from build123d import *

# Parameters (mm, degrees)
SKETCH_1_R               = 7
EXTRUDE_1_DEPTH          = 4
SKETCH_2_R               = 7
EXTRUDE_2_DEPTH          = 30
SKETCH_4_R               = 1
SKETCH_4_R_2             = 0.5
EXTRUDE_3_DEPTH          = 8
EXTRUDE_4_DEPTH          = 4
CUT_EXTRUDE_1_DEPTH      = 4
EXTRUDE_5_DEPTH          = 12
EXTRUDE_5_DEPTH_BACK     = 12
SKETCH_9_R               = 8.062257748
SKETCH_12_R              = 5
CUT_EXTRUDE_2_DEPTH      = 10
CUT_EXTRUDE_3_DEPTH      = 49.277651166
CUT_EXTRUDE_3_DEPTH_BACK = 49.277651166
SKETCH_13_R              = 1.5


with BuildPart() as part:
    # 草图1 → 凸台-拉伸1 (new body)
    with BuildSketch(Plane(origin=(0, 0, 0), x_dir=(1, 0, 0), z_dir=(0, 1, 0))):
        with Locations(Location((0, 0, 0), (0, 0, 270))):
            Circle(SKETCH_1_R)
    extrude(amount=EXTRUDE_1_DEPTH)

    # 草图2 → 凸台-拉伸2 (add)
    with BuildSketch(Plane(origin=(0, 4, 0), x_dir=(1, 0, 0), z_dir=(0, 1, 0))):
        with Locations(Location((0, 0, 0), (0, 0, 270))):
            Circle(SKETCH_2_R)
    extrude(amount=EXTRUDE_2_DEPTH)

    # 草图4 → 凸台-拉伸3 (add)
    with BuildSketch(Plane(origin=(0, 34, 0), x_dir=(1, 0, 0), z_dir=(0, 1, 0))):
        with Locations((5.663466382, -4.114018539)):
            Circle(SKETCH_4_R)
        with Locations((5.663466382, -4.114018539)):
            Circle(SKETCH_4_R_2, mode=Mode.SUBTRACT)
    extrude(amount=-EXTRUDE_3_DEPTH)

    # 草图5 → 凸台-拉伸4 (add)
    with BuildSketch(Plane(origin=(0, 21, 0), x_dir=(-1, 0, 0), z_dir=(0, -1, 0))):
        with BuildLine():
            ThreePointArc((-5.355347766, -4.507798831), (-5.190723909, -4.696422606), (-5.01946017, -4.879038799))
            ThreePointArc((-5.01946017, -4.879038799), (-6.472533008, -4.701735473), (-6.191891648, -3.265038717))
            ThreePointArc((-6.191891648, -3.265038717), (-6.071173774, -3.484372111), (-5.942689761, -3.699248356))
            ThreePointArc((-5.942689761, -3.699248356), (-6.067999695, -4.407877006), (-5.355347766, -4.507798831))
        make_face()
    extrude(amount=EXTRUDE_4_DEPTH)

    # 草图10 → 切除-拉伸1 (cut)
    with BuildSketch(Plane(origin=(0, 34, 0), x_dir=(1, 0, 0), z_dir=(0, 1, 0))):
        with BuildLine():
            ThreePointArc((5.355347766, -4.507798831), (6.067999695, -4.407877006), (5.942689761, -3.699248356))
            ThreePointArc((5.942689761, -3.699248356), (6.071173774, -3.484372111), (6.191891648, -3.265038717))
            ThreePointArc((6.191891648, -3.265038717), (6.472533008, -4.701735473), (5.01946017, -4.879038799))
            ThreePointArc((5.01946017, -4.879038799), (5.190723909, -4.696422606), (5.355347766, -4.507798831))
        make_face()
    extrude(amount=-CUT_EXTRUDE_1_DEPTH, mode=Mode.SUBTRACT)

    # 草图9 → 凸台-拉伸5 (add, two sides: drawn at the far end of the back side and taken through both)
    with BuildSketch(Plane(origin=(0, 0, 0), x_dir=(0, 0, -1), z_dir=(1, 0, 0)).offset(-EXTRUDE_5_DEPTH_BACK)):
        with Locations((0, 38)):
            Circle(SKETCH_9_R)
    extrude(amount=EXTRUDE_5_DEPTH + EXTRUDE_5_DEPTH_BACK)

    # 草图12 → 切除-拉伸2 (cut)
    with BuildSketch(Plane.XZ):
        with Locations(Location((0, 0, 0), (0, 0, 270))):
            Circle(SKETCH_12_R)
    extrude(amount=-CUT_EXTRUDE_2_DEPTH, mode=Mode.SUBTRACT)

    # 草图13 → 切除-拉伸3 (cut, two sides: drawn at the far end of the back side and taken through both)
    with BuildSketch(Plane.XY.offset(-CUT_EXTRUDE_3_DEPTH_BACK)):
        with Locations((0, 6)):
            Circle(SKETCH_13_R)
    extrude(amount=CUT_EXTRUDE_3_DEPTH + CUT_EXTRUDE_3_DEPTH_BACK, mode=Mode.SUBTRACT)


solid = part.part
Geometry: final body of the model. Coordinates: model frame, mm. A direction names the side the tool comes from. Coordinates: 2 decimals unless noted, no trailing zeros. Loops run counter-clockwise (first coordinate to the right, second up) from the corner with the lowest first, then second, coordinate; pieces in that order, holes last. Notation, with made-up numbers: M 37,-11 L 50,-11 A23 cw 50,28 Z; hole C -24,21 d3. An arc over 180 degrees is marked long. One line per item, written item: value. Start each with the question number.
1) Material intervals for L1, parallel to X at y = 4, z = 0; L2, parallel to X at y = 5, z = 4; L3, parallel to Y at x = 0, z = 5.65, sorted ascending. Write a range as from..to.
2) Cut plane D-D (z = -5.75). Return loops of the section in (x, y), then the cut area to 3 significant figures.
3) Reachability of faces 1 (the flat face through (6.2, 26, 4.6)), 2 (the flat face through (0, 10, 0)), 3 (the flat face through (6.2, 17, 4.6)), 4 (the flat face through (5, 0, -2)) from +Z, -Z, +X, -X, +Y, -Y: full face, straight path, thin tool, end or side. Return the list, or none.
4) Cut plane C-C (y = 6). Return loops of the section in (x, z), then the cut area to 3 significant figures.
5) Draft query along X for faces 5 (the flat face through (12, 38, 0)), 6 (the flat face through (6.2, 30, 4.6)), 7 (the cylindrical face through (-1.5, 6.07, -5.9)). Return one class per face: released by +X, released by -X, zero draft, split by the parting line, or undercut.
6) Cut plane B-B (z = 0). Return loops of the section in (x, y), then the cut area to 3 significant figures.
7) Cut plane A-A (x = 0). Return loops of the section in (y, z).
8) Pin query (flat end, axial travel): P1, Ø8, axis at x = 5, y = 31.5, coming from the +Z side; P2, Ø4, axis at y = 6.5, z = -4.5, coming from the -X side; P3, Ø1, axis at x = -5, y = 21, coming from the -Z side; P4, Ø0.5, axis at x = 6, z = 4, coming from the -Y side. Return the tip coordinate at first contact, or that it passes through.
Evaluation:
1. L1: -7..-5, 5..7
1. L2: -5.74..-3, 3..5.74
1. L3: 0..4.5, 7.5..43.75
2. outline: M -12,32.35 L -3.99,32.35 L -3.99,0 L 3.99,0 L 3.99,32.35 L 12,32.35 L 12,43.65 L -12,43.65 Z; hole C 0,6 d3
2. area: 522 mm^2
3. face 1: +Z, +X
3. face 2: -Y
3. face 3: +Z, +X, -Y
3. face 4: +Z, -Z, +X, -X, -Y
4. outline: M -1.5,-6.84 L -1.5,-4.77 A5 cw -1.5,4.77 L -1.5,6.84 A7 ccw Z; M 1.5,-6.84 A7 ccw 1.5,6.84 L 1.5,4.77 A5 cw 1.5,-4.77 Z
4. area: 63.3 mm^2
5. face 5: released by +X
5. face 6: zero draft
5. face 7: undercut
6. outline: M -12,29.94 L -7,29.94 L -7,0 L -5,0 L -5,10 L 5,10 L 5,0 L 7,0 L 7,29.94 L 12,29.94 L 12,46.06 L -12,46.06 Z
6. area: 706 mm^2
7. outline: M 0,-7 L 4.5,-7 L 4.5,-5 L 0,-5 Z; M 0,5 L 4.5,5 L 4.5,7 L 0,7 Z; M 7.5,-7 L 34,-7 A8.06 ccw long 34,7 L 7.5,7 L 7.5,5 L 10,5 L 10,-5 L 7.5,-5 Z
8. P1: z = 7.66
8. P2: x = -6.54
8. P3: z = -5.36
8. P4: y = 0
